Autodesk Inventor part; units mm, degrees
ref_plane "YZ Plane" through (0, 0, 0) normal (1, 0, 0) x (0, 1, 0)
ref_plane "XZ Plane" through (0, 0, 0) normal (0, 1, 0) x (-1, 0, 0)
ref_plane "XY Plane" through (0, 0, 0) normal (0, 0, 1) x (1, 0, 0)
sketch "Boceto2" plane through (0, 0, 0) normal (0, 0, 1) x (1, 0, 0)
  line L0 (130, -85) -> (-130, -85)
  line L1 (-130, -85) -> (-130, 85)
  line L2 (-130, 85) -> (130, 85)
  line L3 (130, 85) -> (130, -85)
  line L4 (130, -85) -> (-130, 85) construction
  line L5 (-130, -85) -> (130, 85) construction
  point P0 (0, 0)
  dimension "d0" = 260
  dimension "d1" = 170
extrude "Extrusión1" add sketch "Boceto2" along normal blind 10
sketch "Boceto3" plane through (0, 0, 10) normal (0, 0, 1) x (1, 0, 0)
  line L0 (-95, 0) -> (-4.19, 0) construction
  circle A0 centre (-95, 0) radius 2.5
  circle A1 centre (-4.19, 0) radius 10
  line L1 (-130, 85) -> (-130, -85)
  line L2 (130, -85) -> (130, 85)
  line L3 (-130, -85) -> (130, -85)
  line L4 (130, 0) -> (80, 0) construction
  line L5 (80, 0) -> (80, -23.2237) construction
  point P0 (0, 0)
  point P1 (-130, 0)
  dimension "d7" = 5
  dimension "d8" = 20
  dimension "d14" = 85
  dimension "d29" = 50
  dimension "d30" = 90.81
  dimension "d31" = 35
  dimension "d32" = 134.19
extrude "Extrusión2" cut sketch "Boceto3" against normal through all
sketch "Boceto5" plane through (0, 0, 0) normal (0, 0, -1) x (-1, 0, 0)
  line L0 (-130, -85) -> (-130, 85)
  line L1 (130, -85) -> (-130, -85)
  line L2 (-130, -85) -> (-130, 85)
  line L3 (-130, 85) -> (130, 85)
  line L4 (130, 85) -> (130, -85)
  line L5 (130, -85) -> (-130, 85) construction
  line L6 (-130, -85) -> (130, 85) construction
  line L7 (119.5, 74.5) -> (-119.5, 74.5)
  line L8 (-119.5, 74.5) -> (-119.5, -74.5)
  line L9 (-119.5, -74.5) -> (119.5, -74.5)
  line L10 (119.5, -74.5) -> (119.5, 74.5)
  circle A0 centre (4.19, 0) radius 10
  circle A1 centre (4.19, 0) radius 20
  circle A2 centre (95, 0) radius 2.5
  circle A3 centre (95, 0) radius 2.5
  point P0 (0, 0)
  dimension "d23" = 10.5
  dimension "d24" = 40
  dimension "d25" = 5
extrude "Extrusión4" add sketch "Boceto5" along normal blind 10 contours L10 L9 L8 L7 | A1
fillet "Empalme1" radius 2 1 edges at (0, -85, 10)
fillet "Empalme2" radius 2 7 edges at (0, 85, 10) (-130, -84.4142, 9.4142) (-130, -85, 4) (-130, 1, 10) (130, -84.4142, 9.4142) (130, -85, 4) (130, 1, 10)
sketch "Boceto6" plane through (0, 0, 10) normal (0, 0, 1) x (1, 0, 0)
  circle A0 centre (-4.19, 0) radius 10
  line L0 (-4.19, 0) -> (35.81, 0)
  line L1 (35.81, 0) -> (35.81, 25)
  line L2 (37.81, 23.5) -> (33.81, 23.5)
  line L3 (33.81, 23.5) -> (33.81, 26.5)
  line L4 (33.81, 26.5) -> (37.81, 26.5)
  line L5 (37.81, 26.5) -> (37.81, 23.5)
  line L6 (37.81, 23.5) -> (33.81, 26.5) construction
  line L7 (33.81, 23.5) -> (37.81, 26.5) construction
  point P0 (0, 0)
  dimension "d35" = 40
  dimension "d36" = 25
  dimension "d38" = 4
  dimension "d39" = 3
extrude "Extrusión5" cut sketch "Boceto6" against normal blind 1.4 contours L2 L3 L4 L5
sketch "Boceto8" plane through (0, 0, 10) normal (0, 0, 1) x (1, 0, 0)
  line L0 (33.81, 23.5) -> (33.81, 26.5)
  line L1 (33.81, 23.5) -> (37.81, 23.5)
  line L2 (37.81, 23.5) -> (37.81, 22.5)
  line L3 (37.81, 22.5) -> (33.81, 22.5)
  line L4 (33.81, 22.5) -> (33.81, 23.5)
  point P0 (0, 0)
  dimension "d42" = 4
  dimension "d43" = 1
extrude "Extrusión6" cut sketch "Boceto8" against normal through all
sketch "Boceto9" plane through (0, 0, 10) normal (0, 0, 1) x (1, 0, 0)
  circle A0 centre (-4.19, 0) radius 10
  circle A1 centre (-4.19, 0) radius 37.5
  circle A2 centre (-4.19, 0) radius 10
  point P0 (0, 0)
  dimension "d47" = 75
extrude "Extrusión7" cut sketch "Boceto9" against normal blind 3
sketch "Boceto10" plane through (0, 0, -10) normal (0, 0, -1) x (-1, 0, 0)
  circle A0 centre (95, 0) radius 2.5
  circle A1 centre (95, 0) radius 18.5
  circle A2 centre (95, 0) radius 6
  point P0 (0, 0)
  dimension "d50" = 37
  dimension "d51" = 12
extrude "Extrusión8" cut sketch "Boceto10" against normal blind 10 contours A1 | A2
sketch "Boceto11" plane through (-95, 0, 0) normal (0, 0, -1) x (-1, 0, 0)
  circle A0 centre (0, 0) radius 2.5
  circle A1 centre (0, 0) radius 6
  point P0 (-95, 0)
  dimension "d54" = 12
extrude "Extrusión9" cut sketch "Boceto11" against normal blind 5
properties part number "Lid"
Could you check a few things on this model? Use its own coordinates, in mm. A direction names the side the tool comes from. Round coordinates to 2 decimals unless told otherwise and drop trailing zeros. Loops run counter-clockwise (first coordinate to the right, second up) from the corner with the lowest first, then second, coordinate; pieces in that order, holes last. Notation, with made-up numbers: (-11.75, -14.75) - (5.25, -14.75) arc R18 ccw to (5.25, 13.25) - close; hole circle Ø2 at (40, 1.25). An arc over 180 degrees is marked (long way). Write item = value, one per line.
1) Imagine slicing it at D-D (x = 111). Please give me the cut outline in (y, z), and give its area (3 significant figures).
Computed:
outline = (-85, 0) - (-74.5, 0) - (-74.5, -10) - (74.5, -10) - (74.5, 0) - (85, 0) - (85, 8) arc R2 ccw to (83, 10) - (-83, 10) arc R2 ccw to (-85, 8) - close
area = 3,190 mm2
2) I need wall thicknesses on line 1 along X through (y, z) = (0.5, -1.5); line 2 along Y through (x, z) = (-4.19, 7.75); line 3 along X through (y, z) = (8, -4.75). Which ranges of each line are inside material? Lowest first, please. Write a range as from..to.
Computed:
line_1 = -119.5..-113.49, -76.51..-14.18, 5.8..119.5
line_2 = -85..-37.5, 37.5..85
line_3 = -119.5..-111.68, -78.32..-10.19, 1.81..119.5
3) Imagine slicing it at B-B (x = -95). Please give me the cut outline in (y, z), and give its area (3 significant figures).
Computed:
outline = (-85, 0) - (-74.5, 0) - (-74.5, -10) - (-18.5, -10) - (-18.5, 0) - (-6, 0) - (-6, 5) - (-2.5, 5) - (-2.5, 10) - (-83, 10) arc R2 ccw to (-85, 8) - close; (2.5, 5) - (6, 5) - (6, 0) - (18.5, 0) - (18.5, -10) - (74.5, -10) - (74.5, 0) - (85, 0) - (85, 8) arc R2 ccw to (83, 10) - (2.5, 10) - close
area = 2,730 mm2
4) Imagine slicing it at A-A (y = 0). Give the number of separate pieces and of enclosed holes in the cut face, and give its area (3 significant figures).
Computed:
separate_pieces = 3
enclosed_holes = 0
area = 3,970 mm2
5) If we mould it in two halves opening along X, with no side actions, what happens to faces 6 (the flat face through (4, -8, 7)), 7 (the flat face through (-130, 0, 4)), 8 (the flat face through (-2, 74.5, -5)), 9 (the flat face through (-90.6, 4.4, 0))? For each: pulls with the +X half, pulls with the -X half, needs draft (parallel to the pull), parting line crosses it, or undercut.
Computed:
face_6 = undercut
face_7 = pulls with the -X half
face_8 = needs draft
face_9 = undercut
6) On a 3-axis mill with a long thin cutter (end or side, diameter ignored), from which of +Z, -Z, +X, -X, +Y, -Y can I reach the whole of each face in a straight line? I mean faces 1 (the cylindrical face through (-9.07, 37.18, 8.52)), 2 (the cylindrical face through (-76.518, 0.813, -5.07)), 3 (the flat face through (2, -74.5, -5)), 4 (the flat face through (-119.5, -1, -5)), 5 (the flat face through (119.5, 1, -5)). Say none if no direction works.
Computed:
face_1 = +Z
face_2 = -Z
face_3 = -Z, +X, -X, -Y
face_4 = -Z, -X, +Y, -Y
face_5 = -Z, +X, +Y, -Y
7) Imagine slicing it at C-C (z = -7). Please give me the cut outline in (x, y).
Computed:
outline = (-119.5, -74.5) - (119.5, -74.5) - (119.5, 74.5) - (-119.5, 74.5) - close; hole circle Ø37 at (-95, 0); hole circle Ø20 at (-4.19, 0); hole (33.81, 22.5) - (37.81, 22.5) - (37.81, 23.5) - (33.81, 23.5) - close
8) I'm going to push flat-ended pins straight in: P1, Ø3, axis at y = -8, z = -7, coming from the +X side; P2, Ø1, axis at x = -79.5, z = -8, coming from the +Y side; P3, Ø2, axis at y = 34.5, z = -7.5, coming from the -X side. Where does each tip first touch, or does it pass through?
Computed:
P1 = 119.5
P2 = 74.5
P3 = -119.5
